from build123d import *

# Parameters (mm, degrees)
SKETCH1_W           = 18
SKETCH1_H           = 100
BOSS_EXTRUDE4_DEPTH = 6
SKETCH1_8_W         = 79
SKETCH1_8_H         = 30
BOSS_EXTRUDE5_DEPTH = 6
CUT_EXTRUDE1_REACH  = 129.581
SKETCH4_W           = 6
SKETCH4_H           = 12


with BuildPart() as part:
    # Sketch1 → Boss-Extrude4 (new body)
    with BuildSketch(Plane.XY):
        with Locations((70, 50)):
            Rectangle(SKETCH1_W, SKETCH1_H)
    extrude(amount=BOSS_EXTRUDE4_DEPTH)

    # Sketch1_8 → Boss-Extrude5 (add)
    with BuildSketch(Plane.XY):
        with Locations((39.5, -15)):
            Rectangle(SKETCH1_8_W, SKETCH1_8_H)
    extrude(amount=BOSS_EXTRUDE5_DEPTH)

    # Sketch4 → Cut-Extrude1 (cut, up to next)
    with BuildSketch(Plane(origin=(0, 0, 0), x_dir=(-1, 0, 0), z_dir=(0, 0, -1)), mode=Mode.PRIVATE) as cut_extrude1_sk1:
        with Locations((-64, 100)):
            Rectangle(SKETCH4_W, SKETCH4_H)
    cut_extrude1_tool1 = extrude(cut_extrude1_sk1.sketch, amount=-CUT_EXTRUDE1_REACH, mode=Mode.PRIVATE) & part.part
    # Sketch4 → Cut-Extrude1 (cut, up to next)
    with BuildSketch(Plane(origin=(0, 0, 0), x_dir=(-1, 0, 0), z_dir=(0, 0, -1)), mode=Mode.PRIVATE) as cut_extrude1_sk2:
        with Locations((-64, 76)):
            Rectangle(SKETCH4_W, SKETCH4_H)
    cut_extrude1_tool2 = extrude(cut_extrude1_sk2.sketch, amount=-CUT_EXTRUDE1_REACH, mode=Mode.PRIVATE) & part.part
    # Sketch4 → Cut-Extrude1 (cut, up to next)
    with BuildSketch(Plane(origin=(0, 0, 0), x_dir=(-1, 0, 0), z_dir=(0, 0, -1)), mode=Mode.PRIVATE) as cut_extrude1_sk3:
        with Locations((-64, 52)):
            Rectangle(SKETCH4_W, SKETCH4_H)
    cut_extrude1_tool3 = extrude(cut_extrude1_sk3.sketch, amount=-CUT_EXTRUDE1_REACH, mode=Mode.PRIVATE) & part.part
    add(cut_extrude1_tool1.solids().sort_by_distance((64, 100, 0))[0], mode=Mode.SUBTRACT)
    add(cut_extrude1_tool2.solids().sort_by_distance((64, 76, 0))[0], mode=Mode.SUBTRACT)
    add(cut_extrude1_tool3.solids().sort_by_distance((64, 52, 0))[0], mode=Mode.SUBTRACT)


solid = part.part
Here's how the part is built. I have some questions about the finished solid (model axes, mm). A direction names the side the tool comes from. Give positions to 0.01 mm unless a question says otherwise; leave off trailing zeros. Loops run counter-clockwise (first coordinate to the right, second up) from the corner with the lowest first, then second, coordinate; pieces in that order, holes last. Notation, with made-up numbers: (58.5, 18) -> (68.5, 18) arc R16 ccw to (68.5, 38) -> close; hole circle Ø1 at (33, -8.75). An arc over 180 degrees is marked (long way). One line per item, written item: value.
Q1. We'd pull the mould along Y, two halves only. Please class faces 4 (the face through (73, 100, 3)), 5 (the face through (64, 70, 3)), 6 (the face through (39, -30, 3)), 7 (the face through (67, 97, 3)): pulls with the +Y half, pulls with the -Y half, needs draft (parallel to the pull), parting line crosses it, or undercut.
Answers follow:
face 4: pulls with the +Y half
face 5: undercut
face 6: pulls with the -Y half
face 7: needs draft
Q2. Suppose I cut it at B-B on y = 77.5. Please give me the cut outline in (x, z).
Answers follow:
outline: (67, 0) -> (79, 0) -> (79, 6) -> (67, 6) -> close
Q3. On a 3-axis mill with a long thin cutter (end or side, diameter ignored), from which of +Z, -Z, +X, -X, +Y, -Y can I reach the whole of each face in a straight line? I mean faces 1 (the face through (65, 7, 6)), 2 (the face through (61, 23, 3)), 3 (the face through (67, 76, 3)). Say none if no direction works.
Answers follow:
face 1: +Z, +X, -X, +Y, -Y
face 2: +Z, -Z, -X, +Y
face 3: +Z, -Z, -X
Q4. I'm going to push flat-ended pins straight in: pin 1 Ø1.8 at (x, z) = (35.5, 1.5) entering from +Y; pin 2 Ø3 at (x, z) = (63.5, 2.5) entering from +Y; pin 3 Ø3 at (y, z) = (98, 4.5) entering from -X. Where does each tip first touch, or does it pass through?
Answers follow:
pin 1: y = 0
pin 2: y = 94
pin 3: x = 67
Q5. If I drill on line 1 along Y through (x, z) = (66, 2.45); line 2 along Y through (x, z) = (27, 2.55); line 3 along X through (y, z) = (93.5, 3.9), over which ranges is the centre line in solid material (lowest first)?
Answers follow:
line 1: -30 to 46, 58 to 70, 82 to 94
line 2: -30 to 0
line 3: 61 to 79
Q6. Suppose I cut it at A-A on z = 3.05. Please give me the cut outline in (x, y), then the cut area to 3 significant figures.
Answers follow:
outline: (0, -30) -> (79, -30) -> (79, 100) -> (67, 100) -> (67, 94) -> (61, 94) -> (61, 82) -> (67, 82) -> (67, 70) -> (61, 70) -> (61, 58) -> (67, 58) -> (67, 46) -> (61, 46) -> (61, 0) -> (0, 0) -> close
area: 3,990 mm^2
Q7. Suppose I cut it at C-C on x = 43.5. Please give me the cut outline in (y, z), then the cut area to 3 significant figures.
Answers follow:
outline: (-30, 0) -> (0, 0) -> (0, 6) -> (-30, 6) -> close
area: 180 mm^2
